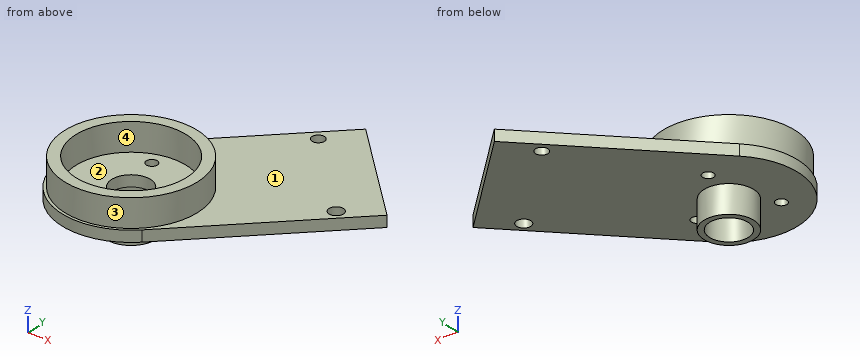
Autodesk Inventor part; units mm, degrees
ref_plane "YZ Plane" through (0, 0, 0) normal (1, 0, 0) x (0, 1, 0)
ref_plane "XZ Plane" through (0, 0, 0) normal (0, 1, 0) x (-1, 0, 0)
ref_plane "XY Plane" through (0, 0, 0) normal (0, 0, 1) x (1, 0, 0)
sketch "Sketch1" plane through (0, 0, 0) normal (0, 0, 1) x (1, 0, 0)
  circle A0 centre (-26.8226, -31.265) radius 3.5
  arc A1 (-35.6614, -22.4261) -> (-17.9837, -40.1038) centre (-26.8226, -31.265) ccw
  circle A2 centre (38.1774, 33.735) radius 1.5
  circle A3 centre (-14.4482, -4.0414) radius 1
  circle A4 centre (0.401, -18.8906) radius 1
  line L0 (-14.4482, -4.0414) -> (0.401, -18.8906)
  line L1 (-17.9837, -40.1038) -> (-35.6614, -22.4261)
  line L2 (-35.6614, -22.4261) -> (-10.9127, 2.3226)
  line L3 (-35.6614, -22.4261) -> (-10.9127, 2.3226)
  line L4 (-10.9127, 2.3226) -> (6.765, -15.3551)
  line L5 (6.765, -15.3551) -> (-17.9837, -40.1038)
  circle A5 centre (-14.4482, -4.0414) radius 1.127
  circle A6 centre (0.401, -18.8906) radius 1.2923
  circle A7 centre (0.401, -18.8906) radius 1.0598
  line L6 (-26.8226, -31.265) -> (-2.0738, -6.5162)
  line L7 (37.1168, 32.6744) -> (38.1774, 33.735)
  point P0 (0, 0)
  point P1 (38.1774, -31.265)
  dimension "d0" = 35
extrude "Extrusion1" add sketch "Sketch1" along normal blind 2 contours A0 L6 L4 L5 L1 | A0 L1 L2 L4 L6 | L1 A1 A0
sketch "Sketch2" plane through (0, 0, 2) normal (0, 0, 1) x (1, 0, 0)
  circle A0 centre (-26.8226, -31.265) radius 3.5
  circle A1 centre (-26.8226, -31.265) radius 10
  circle A2 centre (-26.8226, -31.265) radius 12
  point P0 (0, 0)
  dimension "d3" = 20
  dimension "d4" = 2
extrude "Extrusion2" add sketch "Sketch2" along normal blind 5 contours A2
sketch "Sketch3" plane through (0, 0, 0) normal (0, 0, -1) x (-1, 0, 0)
  line L0 (-6.765, -15.3551) -> (10.9127, 2.3226)
  line L1 (2.0738, -6.5162) -> (35.766, -40.2084)
  circle A0 centre (26.8226, -31.265) radius 3.5
  arc A1 (17.9837, -40.1038) -> (35.6614, -22.4261) centre (26.8226, -31.265) ccw
  line L2 (26.8226, -31.265) -> (17.9837, -40.1038)
  circle A2 centre (32.1259, -36.5683) radius 1
  circle A3 centre (28.7637, -24.0205) radius 1
  circle A4 centre (19.5781, -33.2061) radius 1
  point P0 (0, 0)
  dimension "d7" = 2
  dimension "d8" = 15
  dimension "d11" = 360
extrude "Extrusion3" cut sketch "Sketch3" against normal blind 5 contours A2 L1 | L1 A2 | A3 | A4
sketch "Sketch4" plane through (0, 0, 0) normal (0, 0, -1) x (-1, 0, 0)
  circle A0 centre (32.1259, -36.5683) radius 1
  circle A1 centre (19.5781, -33.2061) radius 1
  circle A2 centre (28.7637, -24.0205) radius 1
  line L0 (17.9837, -40.1038) -> (-6.765, -15.3551)
  arc A3 (17.9837, -40.1038) -> (35.6614, -22.4261) centre (26.8226, -31.265) ccw
  line L1 (10.9127, 2.3226) -> (35.6614, -22.4261)
  line L2 (-6.765, -15.3551) -> (10.9127, 2.3226)
  circle A4 centre (14.4482, -4.0414) radius 1.127
  circle A5 centre (-0.401, -18.8906) radius 1.2923
  circle A6 centre (26.8226, -31.265) radius 3.5
  circle A7 centre (26.8226, -31.265) radius 4.5
  point P0 (0, 0)
  dimension "d15" = 1
extrude "Extrusion4" add sketch "Sketch4" along normal blind 5 contours A7
sketch "Sketch5" plane through (0, 0, 0) normal (1, 0, 0) x (0, 1, 0)
  point P0 (0, 0)
sketch "Sketch6" plane through (0, 0, 0) normal (0, 0, -1) x (-1, 0, 0)
  point P0 (0, 0)
properties part number "motorbracket"
For this review, take the finished solid that the model builds, in its own axes (mm). Face numbers are marked on the shaded views. Round coordinates to 2 decimals unless told otherwise and drop trailing zeros. Loops run counter-clockwise (first coordinate to the right, second up) from the corner with the lowest first, then second, coordinate; pieces in that order, holes last. Notation, with made-up numbers: (87.25, 12.5) - (113.25, 12.5) arc R9 ccw to (113.25, 19.5) - close; hole circle Ø5 at (-8, 21.25). An arc over 180 degrees is marked (long way). Use one line per item in the form item = value.
1) We need section C-C on z = -2.25. Write out the cut boundary in (x, y) (3 decimals), then the cut area to 3 significant figures.
Solutions:
outline = circle Ø9 at (-26.823, -31.265); hole circle Ø7 at (-26.823, -31.265)
area = 25.1 mm2
2) Mouldability with a two-part tool opening along X and no side actions: class the marked faces 1, 2, 3 and 4 as pulls with the +X half, pulls with the -X half, needs draft (parallel to the pull), parting line crosses it, or undercut.
Solutions:
face_1 = needs draft
face_2 = undercut
face_3 = parting line crosses it
face_4 = undercut
3) We need section D-D on y = -14. Write out the cut boundary in (x, z), then the cut area to 3 significant figures.
Solutions:
outline = (-27.24, 0) - (5.41, 0) - (5.41, 2) - (-27.24, 2) - close
area = 65.3 mm2
4) Clearance check with flat-ended pins moving along their axes: P1, Ø6, axis at x = -29.5, y = -30.5, coming from the +Z side; P2, Ø1, axis at y = -36, z = 4.5, coming from the -X side; P3, Ø2.5, axis at x = -19.58, y = -33.21, coming from the -Z side. State where each tip first meets the part, or that it passes through.
Solutions:
P1 = 2
P2 = -38.05
P3 = 0
5) We need section A-A on y = -3.5. Write out the cut boundary in (x, z).
Solutions:
outline = (-16.74, 0) - (-15.44, 0) - (-15.44, 2) - (-16.74, 2) - close; (-13.46, 0) - (-5.09, 0) - (-5.09, 2) - (-13.46, 2) - close
6) Wall thickness on probe 1 along X at (y, z) = (-31, 2.25); probe 2 along X at (y, z) = (-33.5, 1.5); probe 3 along X at (y, z) = (-24, 0.75): over which ranges is each line inside the solid? List them lowest first.
Solutions:
probe_1 = -38.82 to -36.82, -16.83 to -14.83
probe_2 = -39.12 to -29.52, -24.13 to -20.53, -18.62 to -11.38
probe_3 = -36.99 to -29.76, -27.76 to -1.88
7) We need section B-B on x = -32. Write out the cut boundary in (y, z), then the cut area to 3 significant figures.
Solutions:
outline = (-42.64, 0) - (-37.56, 0) - (-37.56, 2) - (-39.82, 2) - (-39.82, 7) - (-42.09, 7) - (-42.09, 2) - (-42.64, 2) - close; (-35.58, 0) - (-18.76, 0) - (-18.76, 2) - (-20.44, 2) - (-20.44, 7) - (-22.71, 7) - (-22.71, 2) - (-35.58, 2) - close
area = 66.5 mm2
